from build123d import *

# Parameters (mm, degrees)
SKETCH1_R               = 4
BOSS_EXTRUDE3_DEPTH     = 3.4
BOSS_EXTRUDE5_START     = 0.5
SKETCH3_R               = 4
BOSS_EXTRUDE5_DEPTH     = 0.5
BOSS_EXTRUDE6_DEPTH     = 0.5
SKETCH8_R               = 0.125
BOSS_EXTRUDE10_DEPTH    = 1.5
SKETCH9_R               = 0.0625
SKETCH9_R_2             = 0.065
BOSS_EXTRUDE11_DEPTH    = 1
CONG_1_R                = 1
ESQUISSE1_R             = 3.7
ESQUISSE1_R_2           = 3.4
ENL_V_MAT_EXTRU_1_DEPTH = 0.2


with BuildPart() as part:
    # Sketch1 → Boss-Extrude3 (new body)
    with BuildSketch(Plane(origin=(0, 0, 0), x_dir=(1, 0, 0), z_dir=(0, 1, 0))):
        with Locations(Location((2.012990556, 4.989015145, 0), (0, 0, 270))):
            Circle(SKETCH1_R)
    extrude(amount=-BOSS_EXTRUDE3_DEPTH)

    # Sketch3 → Boss-Extrude5 (add)
    with BuildSketch(Plane(origin=(0, 0, 0), x_dir=(1, 0, 0), z_dir=(0, 1, 0)).offset(BOSS_EXTRUDE5_START)):
        with Locations(Location((2.012990556, 4.989015145, 0), (0, 0, 270))):
            Circle(SKETCH3_R)
    extrude(amount=-BOSS_EXTRUDE5_DEPTH)

    # Sketch5 → Boss-Extrude6 (add)
    with BuildSketch(Plane(origin=(0, 0.5, 0), x_dir=(1, 0, 0), z_dir=(0, 1, 0))):
        with BuildLine():
            ThreePointArc((3.512990556, 1.280915901), (2.012990556, 0.989015145), (0.512990556, 1.280915901))
            Line((0.512990556, 1.280915901), (0.512990556, -2.010984855))
            Line((0.512990556, -2.010984855), (3.512990556, -2.010984855))
            Line((3.512990556, -2.010984855), (3.512990556, 1.280915901))
        make_face()
    extrude(amount=-BOSS_EXTRUDE6_DEPTH)

    # Sketch8 → Boss-Extrude10 (add)
    with BuildSketch(Plane.XY.offset(2.010984855)):
        with Locations((2.334197454, 0)):
            Circle(SKETCH8_R)
        with Locations((1.65473302, 0)):
            Circle(SKETCH8_R)
    extrude(amount=BOSS_EXTRUDE10_DEPTH)

    # Sketch9 → Boss-Extrude11 (add)
    with BuildSketch(Plane.XY.offset(3.510984855)):
        with Locations((2.332150334, 0)):
            Circle(SKETCH9_R)
        with Locations((1.65473302, 0)):
            Circle(SKETCH9_R_2)
    extrude(amount=BOSS_EXTRUDE11_DEPTH)

    # Congé1
    # the kernel refuses this fillet: 1 mm, written as the material it adds along each edge
    with BuildSketch(Plane(origin=(-0.290802546, 0, 2.010984855), x_dir=(0, 0, -1), z_dir=(1, 0, 0))) as cong_1_piece_1_section:
        with BuildLine():
            CenterArc((CONG_1_R, -CONG_1_R), CONG_1_R, 90, 90)
            Line((0, -CONG_1_R), (0, 0))
            Line((0, 0), (CONG_1_R, 0))
        make_face()
    cong_1_piece_1 = extrude(amount=5.25, mode=Mode.PRIVATE)
    cong_1_piece_1 = cong_1_piece_1 & Plane(origin=(2.334197454, 0, 1.652352457), x_dir=(1, 0, 0), z_dir=(0, 0, -1)) * Cylinder(0.125, 15, mode=Mode.PRIVATE)
    add(cong_1_piece_1)
    with BuildSketch(Plane(origin=(-0.290802546, 0, 2.010984855), x_dir=(0, 0, -1), z_dir=(1, 0, 0))) as cong_1_piece_2_section:
        with BuildLine():
            CenterArc((CONG_1_R, -CONG_1_R), CONG_1_R, 90, 90)
            Line((0, -CONG_1_R), (0, 0))
            Line((0, 0), (CONG_1_R, 0))
        make_face()
    cong_1_piece_2 = extrude(amount=5.25, mode=Mode.PRIVATE)
    cong_1_piece_2 = cong_1_piece_2 & Plane(origin=(1.65473302, 0, 1.652352457), x_dir=(1, 0, 0), z_dir=(0, 0, -1)) * Cylinder(0.125, 15, mode=Mode.PRIVATE)
    add(cong_1_piece_2)
    with BuildSketch(Plane(origin=(-0.97026698, 0, 2.010984855), x_dir=(0, 0, -1), z_dir=(1, 0, 0))) as cong_1_piece_3_section:
        with BuildLine():
            CenterArc((CONG_1_R, -CONG_1_R), CONG_1_R, 90, 90)
            Line((0, -CONG_1_R), (0, 0))
            Line((0, 0), (CONG_1_R, 0))
        make_face()
    cong_1_piece_3 = extrude(amount=5.25, mode=Mode.PRIVATE)
    cong_1_piece_3 = cong_1_piece_3 & Plane(origin=(2.334197454, 0, 1.652352457), x_dir=(1, 0, 0), z_dir=(0, 0, -1)) * Cylinder(0.125, 15, mode=Mode.PRIVATE)
    add(cong_1_piece_3)
    with BuildSketch(Plane(origin=(-0.97026698, 0, 2.010984855), x_dir=(0, 0, -1), z_dir=(1, 0, 0))) as cong_1_piece_4_section:
        with BuildLine():
            CenterArc((CONG_1_R, -CONG_1_R), CONG_1_R, 90, 90)
            Line((0, -CONG_1_R), (0, 0))
            Line((0, 0), (CONG_1_R, 0))
        make_face()
    cong_1_piece_4 = extrude(amount=5.25, mode=Mode.PRIVATE)
    cong_1_piece_4 = cong_1_piece_4 & Plane(origin=(1.65473302, 0, 1.652352457), x_dir=(1, 0, 0), z_dir=(0, 0, -1)) * Cylinder(0.125, 15, mode=Mode.PRIVATE)
    add(cong_1_piece_4)

    # Esquisse1 → Enlèv. mat.-Extru.1 (cut)
    with BuildSketch(Plane(origin=(0, 0.5, 0), x_dir=(1, 0, 0), z_dir=(0, 1, 0))):
        with Locations(Location((2.012990556, 4.989015145, 0), (0, 0, 270))):
            Circle(ESQUISSE1_R)
        with Locations(Location((2.012990556, 4.989015145, 0), (0, 0, 270))):
            Circle(ESQUISSE1_R_2, mode=Mode.SUBTRACT)
    extrude(amount=-ENL_V_MAT_EXTRU_1_DEPTH, mode=Mode.SUBTRACT)


solid = part.part
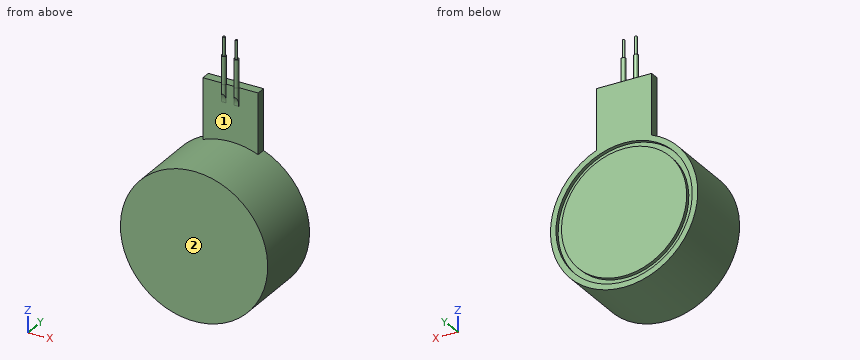
Here's how the part is built. I have some questions about the finished solid (model axes, mm). Face numbers are marked on the shaded views. A direction names the side the tool comes from. Coordinates: 2 decimals unless noted, no trailing zeros. Write each loop counter-clockwise with the first axis right and the second up, starting at its lowest first coordinate (ties: lowest second). Pieces come first, ordered by that corner, then holes.
1) If we section it at D-D (y = -1.85): List the corners of the cut face in (x, z) for me, plus the area to 3 significant figures.
Filled in:
outline: circle Ø8 at (2.01, -4.99)
area: 50.3 mm2
2) If we section it at A-A (z = 2.5): List the corners of the cut face in (x, y) for me (3 decimals).
Filled in:
outline: circle Ø0.25 at (1.655, 0); circle Ø0.25 at (2.334, 0)
3) If we section it at C-C (z = -4): List the corners of the cut face in (x, y) for me.
Filled in:
outline: (-1.86, -3.4) - (5.89, -3.4) - (5.89, 0.5) - (5.58, 0.5) - (5.58, 0.3) - (5.27, 0.3) - (5.27, 0.5) - (-1.24, 0.5) - (-1.24, 0.3) - (-1.55, 0.3) - (-1.55, 0.5) - (-1.86, 0.5) - close
4) Which directions (+Z, -Z, +X, -X, +Y, -Y) give clear straight access to the entire face, cutting with the end or side of a thin tool? Please do the marked faces 1 and 2.
Filled in:
face 1: -Y
face 2: +Z, -Z, +X, -X, -Y
5) If we section it at B-B (x = 4): List the corners of the cut face in (y, z) for me, plus the area to 3 significant figures.
Filled in:
outline: (-3.4, -8.46) - (0.5, -8.46) - (0.5, -8.11) - (0.3, -8.11) - (0.3, -7.75) - (0.5, -7.75) - (0.5, -2.23) - (0.3, -2.23) - (0.3, -1.87) - (0.5, -1.87) - (0.5, -1.52) - (-3.4, -1.52) - close
area: 26.9 mm2
6) If I drill on line 1 (Y direction, x = 5.25, z = -3.5); line 2 (Y direction, x = 2, z = 1.75); line 3 (Z direction, x = 0.5, y = -0.95), over which ranges is the centre line in solid material (lowest first)?
Filled in:
line 1: y = -3.4 to 0.3
line 2: y = 0 to 0.5
line 3: z = -8.69 to -1.29
7) I'm going to push flat-ended pins straight in: pin 1 (1.5 mm diameter, centred on x = -1, y = 0, fed in from +Z); pin 2 (0.9 mm diameter, centred on x = 2, z = -0.5, fed in from -Y). Where does each tip first touch, or does it pass through?
Filled in:
pin 1: stops at z = -1.69
pin 2: stops at y = 0
